from build123d import *

# Parameters (mm, degrees)
F0_R     = 1.5
F1_DEPTH = 3
F2_SIZE  = 3.99999


# Not quite as in the source:
# - a fillet or chamfer is up to 0.001 mm smaller than in the source, because OpenCascade refuses the exact size


with BuildPart() as f1:
    # F0 (on Front) → F1 (new body)
    with BuildSketch(Plane.XZ):
        with BuildLine():
            Line((5.6, -62), (5.6, 12))
            ThreePointArc((5.6, 12), (0, 17.6), (-5.6, 12))
            Line((-5.6, 12), (-5.6, -62))
            Line((-5.6, -62), (-1.6, -62))
            Line((-1.6, -62), (-1.6, -49))
            Line((-1.6, -49), (1.6, -49))
            Line((1.6, -49), (1.6, -62))
            Line((1.6, -62), (5.6, -62))
        make_face()
        with Locations((0, -14)):
            Circle(F0_R, mode=Mode.SUBTRACT)
        with BuildLine():
            ThreePointArc((1.6, 0), (0, -1.6), (-1.6, 0))
            Line((-1.6, 0), (-1.6, 12))
            ThreePointArc((-1.6, 12), (0, 13.6), (1.6, 12))
            Line((1.6, 12), (1.6, 0))
        make_face(mode=Mode.SUBTRACT)
    extrude(amount=F1_DEPTH)

    # F2 (size 4 in the source; OpenCascade refuses exactly that, so slightly less here)
    f2_edges = [f1.edges().sort_by_distance(p)[0] for p in [
        (5.6, -1.5, -62),
        (-5.6, -1.5, -62),
    ]]
    chamfer(f2_edges, length=F2_SIZE)


solid = f1.part
Input: part model. Units: mm. Frame: model coordinates. A direction names the side the tool comes from. Round coordinates to 2 decimals unless told otherwise and drop trailing zeros. Loops run counter-clockwise (first coordinate to the right, second up) from the corner with the lowest first, then second, coordinate; pieces in that order, holes last. Notation, with made-up numbers: (-19, -25.75) -> (7, -25.75) arc R28 cw to (7, -4.75) -> close; hole circle Ø11 at (-12.5, 60.5). An arc over 180 degrees is marked (long way). Answer as a JSON object with one key per item and string values. Group by question number.
1) Draft query along X for faces 4 (the cylindrical face through (0, -1.5, -1.6)), 5 (the flat face through (5.6, -1, -23)), 6 (the cylindrical face through (0.1, -1.5, 17.6)), 7 (the cylindrical face through (-0.325, -1.479, -15.464)). Return one class per face: +X half, -X half, draft (parallel to the pull), parting line (faces both ways), or undercut.
2) Section query A-A on x = 0. Output: boundary loops of the cut face in (y, z).
3) Pin query (flat end, axial travel): pin 1 (1.5 mm diameter, centred on x = 0.5, y = -1, fed in from -Z); pin 2 (1.5 mm diameter, centred on x = -3, y = -1.5, fed in from +Z). Return the tip coordinate at first contact, or that it passes through.
4) Section query C-C on y = -2. State how many separate pieces and enclosed holes the cut face has, plus the area to 3 significant figures.
5) Section query D-D on z = 1.5. Output: boundary loops of the cut face in (x, y).
6) Ray query, L1, parallel to Z at x = 0, y = -1.65; L2, parallel to X at y = -0.5, z = 9.5; L3, parallel to Z at x = 1.25, y = -0.85. Return the intervals inside material, ascending.
7) Reachability of faces 1 (the flat face through (0, -1, -49)), 2 (the cylindrical face through (0, -1.5, 13.6)), 3 (the flat face through (0, 0, -22)) from +Z, -Z, +X, -X, +Y, -Y: full face, straight path, thin tool, end or side. Return the list, or none.
8) Section query B-B on z = -14. Output: boundary loops of the cut face in (x, y), plus the area to 3 significant figures.
Reply:
{
 "1": {"face 4": "undercut", "face 5": "+X half", "face 6": "parting line", "face 7": "undercut"},
 "2": {"outline": "(-3, -49) -> (0, -49) -> (0, -15.5) -> (-3, -15.5) -> close; (-3, -12.5) -> (0, -12.5) -> (0, -1.6) -> (-3, -1.6) -> close; (-3, 13.6) -> (0, 13.6) -> (0, 17.6) -> (-3, 17.6) -> close"},
 "3": {"pin 1": "stops at z = -49", "pin 2": "stops at z = 17.13"},
 "4": {"separate pieces": "1", "enclosed holes": "2", "area": "767 mm2"},
 "5": {"outline": "(-5.6, -3) -> (-1.6, -3) -> (-1.6, 0) -> (-5.6, 0) -> close; (1.6, -3) -> (5.6, -3) -> (5.6, 0) -> (1.6, 0) -> close"},
 "6": {"L1": "z = -49 to -15.5, -12.5 to -1.6, 13.6 to 17.6", "L2": "x = -5.6 to -1.6, 1.6 to 5.6", "L3": "z = -49 to -14.83, -13.17 to -1, 13 to 17.46"},
 "7": {"face 1": "-Z, +Y, -Y", "face 2": "+Y, -Y", "face 3": "+Z, -Z, +X, -X, +Y"},
 "8": {"outline": "(-5.6, -3) -> (-1.5, -3) -> (-1.5, 0) -> (-5.6, 0) -> close; (1.5, -3) -> (5.6, -3) -> (5.6, 0) -> (1.5, 0) -> close", "area": "24.6 mm2"}
}
